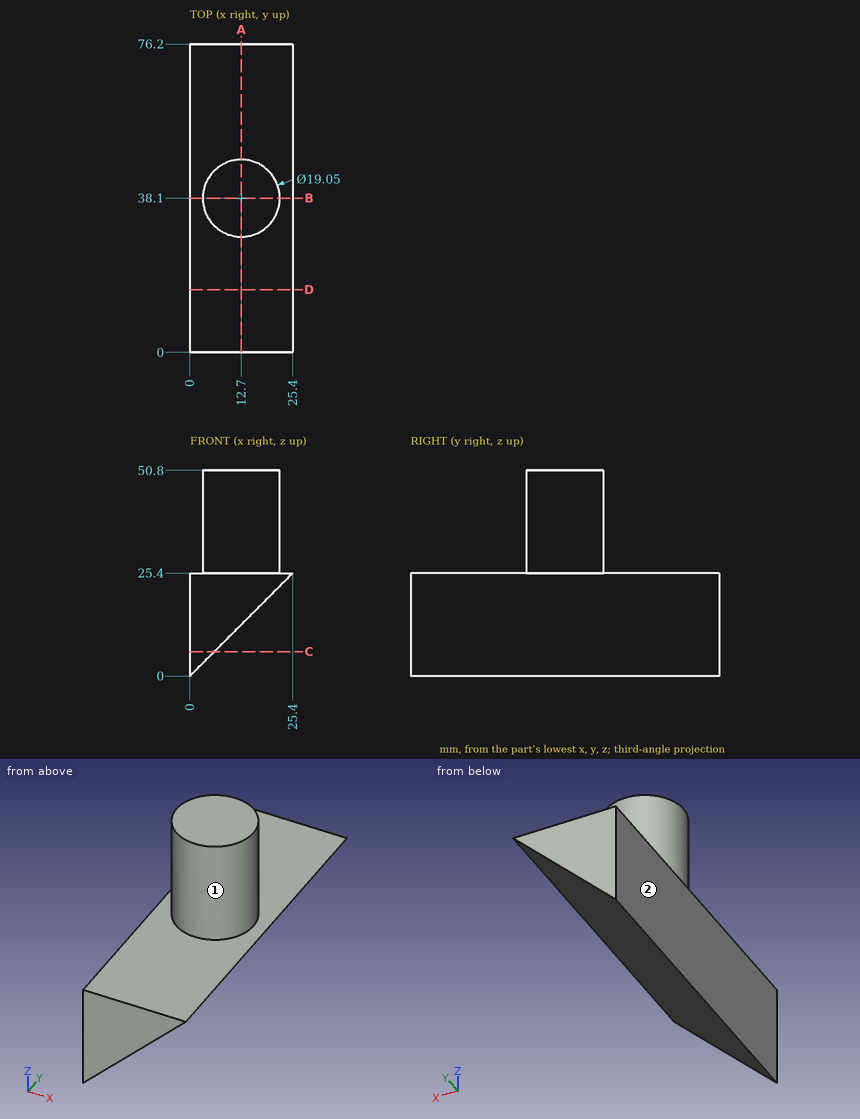
Could you check a few things on this drawing? It's one solid part, dimensions in mm from its lowest x, y, z. A direction names the side the tool comes from. Give positions to 0.01 mm unless a question says otherwise; leave off trailing zeros. Order: outer loops, then holes, each group sorted by start corner. A loop starts at its lowest first (then second) coordinate and runs counter-clockwise, first axis right, second up. Notation, with made-up numbers: (24.25, -17) - (72.25, -17) arc R17 cw to (72.25, -12) - close; hole circle Ø3 at (49.25, 51.5). An arc over 180 degrees is marked (long way). Answer as a JSON object with one key per item and string values. Group by question number.
Item 1: Please list where these lines run through material, in increasing order: probe 1 along X at (y, z) = (14.5, 23); probe 2 along Y at (x, z) = (17.5, 41); probe 3 along X at (y, z) = (71.5, 4).
Item 2: If we section it at C-C on z = 6: Please give me the cut outline in (x, y), and give its area (3 significant figures).
Item 3: If we section it at D-D on y = 15.5: Please give me the cut outline in (x, z).
Item 4: If we section it at B-B on y = 38.1: Please give me the cut outline in (x, z) (3 decimals).
Item 5: If we section it at A-A on x = 12.7: Please give me the cut outline in (y, z) (3 decimals), and give its area (3 significant figures).
Item 6: For P1, Ø7.5, axis at x = 10.5, y = 20, coming from the +Z side; P2, Ø3, axis at x = 14.5, y = 13.5, coming from the -Z side; P3, Ø2, axis at x = 13.5, y = 43.5, coming from the -Z side, each with a flat end and sliding along its axis, tell me the tip position at first contact or that it passes through.
Item 7: Which directions (+Z, -Z, +X, -X, +Y, -Y) give clear straight access to the entire face, cutting with the end or side of a thin tool? Please do the marked faces 1 and 2.
Result set:
{
 "1": {"probe 1": "0 to 23", "probe 2": "29.87 to 46.33", "probe 3": "0 to 4"},
 "2": {"outline": "(0, 0) - (6, 0) - (6, 76.2) - (0, 76.2) - close", "area": "457 mm²"},
 "3": {"outline": "(0, 0) - (25.4, 25.4) - (0, 25.4) - close"},
 "4": {"outline": "(0, 0) - (25.4, 25.4) - (22.225, 25.4) - (22.225, 50.8) - (3.175, 50.8) - (3.175, 25.4) - (0, 25.4) - close"},
 "5": {"outline": "(0, 12.7) - (76.2, 12.7) - (76.2, 25.4) - (47.625, 25.4) - (47.625, 50.8) - (28.575, 50.8) - (28.575, 25.4) - (0, 25.4) - close", "area": "1,450 mm²"},
 "6": {"P1": "z = 25.4", "P2": "z = 13", "P3": "z = 12.5"},
 "7": {"face 1": "+Z", "face 2": "+Z, -Z, -X, +Y, -Y"}
}
